Part model, mm, in its own coordinate system. Face numbers are marked on the shaded views. A direction names the side the tool comes from. Give positions to 0.01 mm unless a question says otherwise; leave off trailing zeros. Write each loop counter-clockwise with the first axis right and the second up, starting at its lowest first coordinate (ties: lowest second). Pieces come first, ordered by that corner, then holes. Notation, with made-up numbers: M 89.25,73 L 132.25,73 A20 ccw 132.25,98 Z; hole C 12.5,-4.75 d7. An arc over 180 degrees is marked long. Use CSV: the item, a comma, the result in double quotes. Start each with the question number.
Item 1: Cut at A-A (y = 9). List the corners of the cut face in (x, z).
Item 2: Which spindle directions (+Z, -Z, +X, -X, +Y, -Y) get a long thin tool onto all of the face, cutting with end or side? Do the marked faces 1, 2 and 3. Say none if no direction does.
Item 3: Drill centre lines: line 1 (Z direction, x = 2.5, y = -4.5); line 2 (X direction, y = -5.25, z = 6.5); line 3 (Z direction, x = 0, y = 8.7). Where is each one in solid material? Low to high. Write a range as [from, to].
Item 4: Mould opens along Y. For the marked faces 4, 5 and 6 say: released by +Y, released by -Y, zero draft, split by the parting line, or undercut.
Item 5: Cut at B-B (z = 19). List the corners of the cut face in (x, y), then the cut area to 3 significant figures.
Item 6: Cut at C-C (y = 2.75). List the corners of the cut face in (x, z).
Item 7: Pin check, flat tips, straight feed: pin 1 (9.5 mm diameter, centred on x = 0, z = 0, fed in from -Y); pin 2 (3 mm diameter, centred on x = -15, y = 7.5, fed in from +Z); pin 3 (6 mm diameter, centred on y = -11, z = -15.5, fed in from +X); pin 4 (14 mm diameter, centred on x = -10.5, z = 11.5, fed in from -Y). Stop position of each tip, or through.
Item 8: Cut at D-D (y = -3.5). List the corners of the cut face in (x, z).
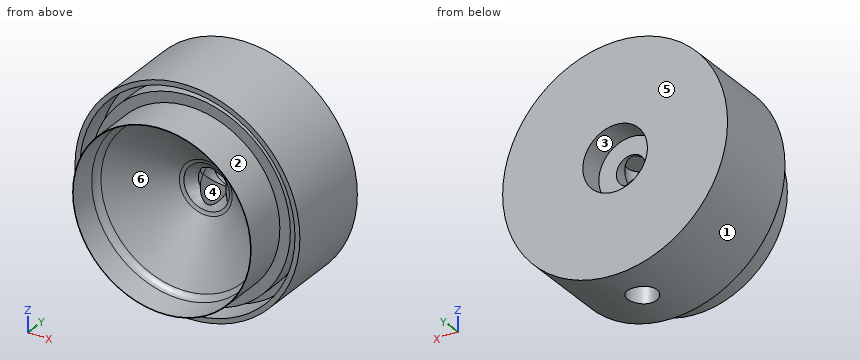
Autodesk Inventor part; units mm, degrees
ref_plane "YZ Plane" through (0, 0, 0) normal (1, 0, 0) x (0, 1, 0)
ref_plane "XZ Plane" through (0, 0, 0) normal (0, 1, 0) x (-1, 0, 0)
ref_plane "XY Plane" through (0, 0, 0) normal (0, 0, 1) x (1, 0, 0)
sketch "Sketch1" plane through (0, 0, 0) normal (0, 0, 1) x (1, 0, 0)
  line L0 (3, 12) -> (23, 12)
  line L1 (23, 12) -> (23, 0)
  line L2 (3, 2) -> (3, 12)
  line L3 (0, 19.5472) -> (0, -22.4151)
  line L4 (23, 0) -> (22, 0) construction
  line L5 (22, 0) -> (22, -6)
  line L6 (22, -6) -> (23, -6)
  line L7 (23, -6) -> (23, 0)
  line L8 (20.4, 0) -> (17.25, 0) construction
  line L9 (17.25, 0) -> (17.25, -5) construction
  line L10 (17.25, -5) -> (20.4, -5) construction
  line L11 (20.4, -5) -> (20.4, 0)
  arc A0 (3, 2) -> (4.6637, 0.0285) centre (5, 2) ccw
  line L12 (22, 0) -> (20.4, 0)
  line L13 (17.25, 0) -> (5, 0)
  line L14 (-20.0393, 0) -> (22, 0) construction
  line L15 (23, 0) -> (24.5476, 0) construction
  line L16 (18.25, 0) -> (18.25, -5) construction
  line L17 (20.4, -5) -> (18.25, -5)
  line L18 (18.25, -5) -> (18.25, -14)
  line L19 (18.25, -14) -> (18.15, -14)
  line L20 (18.15, -14) -> (17.25, -5) construction
  line L21 (18.25, -8) -> (17.55, -8) construction
  line L22 (5.4025, -0.2566) -> (16.7316, -7.4783)
  line L23 (17.6466, -8.9658) -> (18.15, -14)
  arc A1 (17.6466, -8.9658) -> (16.7316, -7.4783) centre (15.6565, -9.1648) ccw
  arc A2 (5.4025, -0.2566) -> (4.6637, 0.0285) centre (4.3274, -1.943) ccw
  point P0 (0, 0)
  point P1 (17.25, 0)
  point P2 (17.25, -5)
  point P3 (5, 0)
  point P4 (17.9, -8)
  dimension "d0" = 6
  dimension "d2" = 1
  dimension "d5" = 5
  dimension "d6" = 1.6
  dimension "d7" = 44
  dimension "d11" = 2
  dimension "d12" = 12
  dimension "d14" = 6
  dimension "d23" = 36.5
  dimension "d24" = 1
  dimension "d25" = 0.1
  dimension "d26" = 9
  dimension "d37" = 3
  dimension "d38" = 2
  dimension "d39" = 2
revolve "Revolution1" add sketch "Sketch1" angle 360 about axis through (0, 19.5472, 0) along (0, -1, 0)
sketch "Sketch2" plane through (0, 0, 0) normal (0, 0, 1) x (1, 0, 0)
  line L0 (-3, 12) -> (3, 12)
  line L1 (0, 12) -> (0, 0) construction
  line L2 (-3, 2) -> (3, 2) construction
  circle A0 centre (0, 3.5) radius 3
  line L3 (-20.4, 0) -> (20.4, 0)
  point P0 (2.5981, 2)
  point P1 (-2.5981, 2)
  dimension "d0" = 6
  dimension "d16" = 6
  dimension "d40" = 3.5
extrude "Extrusion1" cut sketch "Sketch2" along normal blind 3 and the other way blind 33
sketch "Sketch3" plane through (0, 12, 0) normal (0, 1, 0) x (1, 0, 0)
  circle A0 centre (0, 0) radius 6.6
  circle A1 centre (0, 0) radius 3 construction
  dimension "d0" = 6
  dimension "d27" = 13.2
extrude "Extrusion2" cut sketch "Sketch3" against normal blind 5
equation "\"d0\" = t_D"
equation "\"d2\" = w_th"
equation "\"d5\" = b_rim_h"
equation "\"d6\" = lv_th"
equation "\"d7\" = b_OD"
equation "\"d11\" = fillet_D"
equation "\"d12\" = top_th_f"
equation "\"d14\" = w_l"
equation "\"d23\" = b_ID"
equation "\"d24\" = w_th"
equation "\"d25\" = tol"
equation "\"d26\" = 1.5 * w_l"
equation "\"d38\" = fillet_D"
equation "\"d39\" = fillet_D"
equation "\"d16\" = t_D"
equation "\"d40\" = 0.5 * w_th + 0.5 * t_D"
equation "\"d18\" = 0.5 * t_D"
equation "\"d19\" = 0.75 * b_OD"
equation "\"d27\" = cn_D"
equation "\"d30\" = cn_h"
equation "\"tol\" = 0.1"
equation "\"fillet_D\" = 2"
equation "\"w_th\" = 1"
equation "\"w_l\" = 6"
equation "\"t_D\" = 6"
equation "\"t_D_f\" = t_D + w_th"
equation "\"top_th_f\" = t_D_f + cn_h"
equation "\"cn_h\" = 5"
equation "\"lv_th\" = 1.6"
equation "\"d3\" = w_l"
equation "\"d8\" = top_th_f"
equation "\"b_ID\" = 36.5"
equation "\"b_OD\" = 44"
equation "\"b_rim_h\" = 5"
equation "\"top_th\" = t_D + w_th"
equation "\"lv_OD\" = 26"
equation "\"sv_OD\" = 13"
equation "\"sv_th\" = 1.5"
equation "\"b_th\" = 1.5"
equation "\"h_s\" = 2.25"
equation "\"h_D\" = 0.9"
equation "\"v_h_D\" = 7.5"
equation "\"v_h_off\" = 0.5 * cn_D + 0.5 * v_h_D"
properties part number "bottle"
Worked answers:
1,outline,"C 0,0 d46; hole C 0,0 d13.2"
2,face 1,"+Y, -Y"
2,face 2,"-Y"
2,face 3,"+Y"
3,line 1,"z = [-22.86, -21.86], [-20.25, -11.8], [11.8, 20.25], [21.86, 22.86]"
3,line 2,"x = [-22.06, -21.02], [-17.05, -11.53], [11.53, 17.05], [21.02, 22.06]"
3,line 3,"z = [-23, -6.6], [6.6, 23]"
4,face 4,"undercut"
4,face 5,"released by +Y"
4,face 6,"released by -Y"
5,outline,"M -12.96,-6 L -11.09,-6 L -11.09,0 L -7.43,0 L -7.43,-5 L 7.43,-5 L 7.43,0 L 11.09,0 L 11.09,-6 L 12.96,-6 L 12.96,12 L -12.96,12 Z"
5,area,"408 mm^2"
6,outline,"M -2.9,-22.82 L -2.9,-0.75 A3 cw -2.9,0.75 L -2.9,3 L 2.9,3 L 2.9,0.75 A3 cw 2.9,-0.75 L 2.9,-22.82 A23 ccw long Z"
7,pin 1,"stops at y = 0.01"
7,pin 2,"stops at z = 18.62"
7,pin 3,"stops at x = 13.3"
7,pin 4,"stops at y = -14"
8,outline,"C 0,0 d46; C 0,0 d40.8; hole C 0,0 d44; hole C 0,0 d20.98"
